Input: dimensioned drawing with shaded views. Units: mm. Origin: part minimum x, y, z. Round coordinates to 2 decimals unless told otherwise and drop trailing zeros. Loops run counter-clockwise (first coordinate to the right, second up) from the corner with the lowest first, then second, coordinate; pieces in that order, holes last. Notation, with made-up numbers: (-14.75, 35.25) -> (23.25, 35.25) arc R21 cw to (23.25, 50.25) -> close; hole circle Ø2 at (-22.75, 1). An arc over 180 degrees is marked (long way). Answer as a JSON object with one key per item and string values.
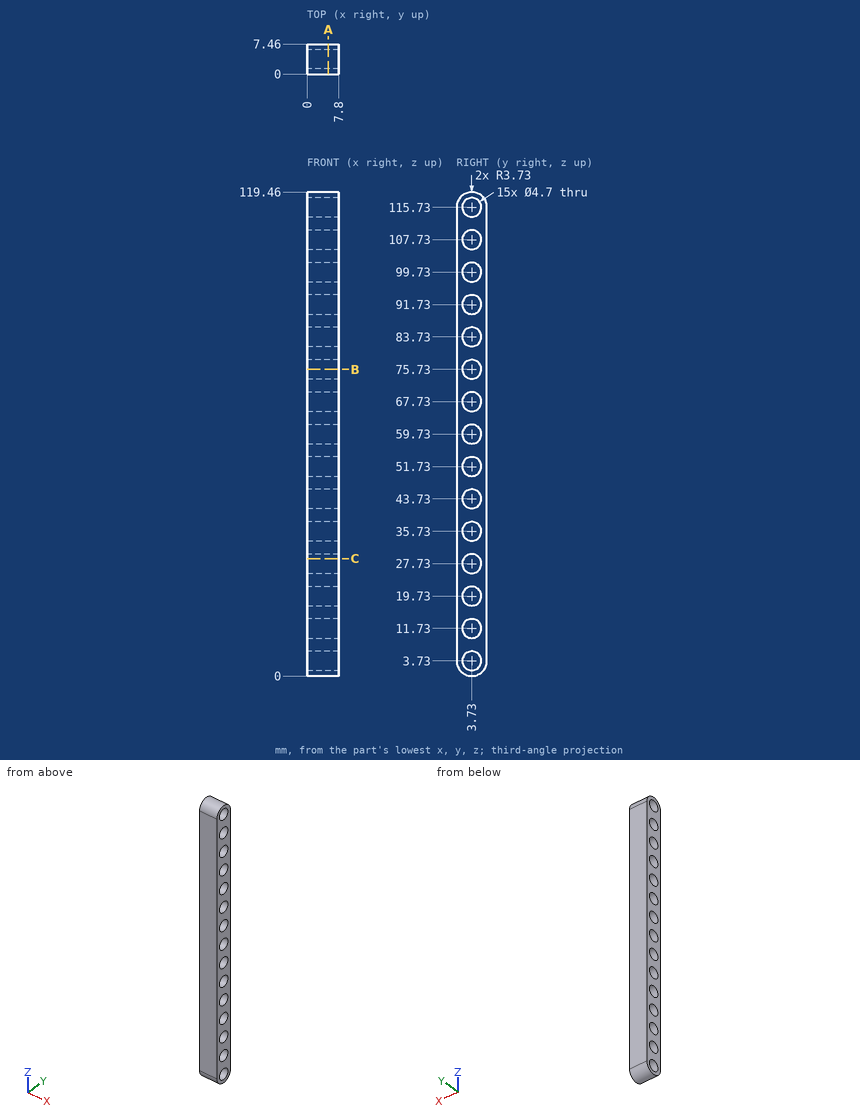
1) Section C-C, the plane z = 29. Output: boundary loops of the cut face in (x, y), plus the area to 3 significant figures.
Output:
{"outline": "(0, 0) -> (7.8, 0) -> (7.8, 1.75) -> (0, 1.75) -> close; (0, 5.71) -> (7.8, 5.71) -> (7.8, 7.46) -> (0, 7.46) -> close", "area": "27.3 mm^2"}
2) Contact query for flat-ended pins moving along their axis: P1, Ø4, axis at x = 4, y = 1, coming from the +Z side; P2, Ø4, axis at y = 3.73, z = 91.73, coming from the -X side. Output: stop coordinate, or through.
Output:
{"P1": "stops at z = 119.39", "P2": "passes through"}
3) Section B-B, the plane z = 75.73. Output: boundary loops of the cut face in (x, y).
Output:
{"outline": "(0, 0) -> (7.8, 0) -> (7.8, 1.38) -> (0, 1.38) -> close; (0, 6.08) -> (7.8, 6.08) -> (7.8, 7.46) -> (0, 7.46) -> close"}
4) Ray query, probe 1 along Y at (x, z) = (2.5, 67.73); probe 2 along Y at (x, z) = (5.75, 10); probe 3 along Z at (x, y) = (1.75, 6.75). Return the intervals inside material, ascending.
Output:
{"probe 1": "y = 0 to 1.38, 6.08 to 7.46", "probe 2": "y = 0 to 2.14, 5.32 to 7.46", "probe 3": "z = 1.54 to 117.92"}
5) Section A-A, the plane x = 5.25. Count the separate pieces of the cut face and the enclosed holes in it, plus the area to 3 significant figures.
Output:
{"separate pieces": "1", "enclosed holes": "15", "area": "619 mm^2"}
